Check sheet for the modelled part. Datum: model origin and axes. Units: mm. A direction names the side the tool comes from. Round coordinates to 2 decimals unless told otherwise and drop trailing zeros. Loops run counter-clockwise (first coordinate to the right, second up) from the corner with the lowest first, then second, coordinate; pieces in that order, holes last. Notation, with made-up numbers: (12, 32.25) -> (65, 32.25) arc R12 ccw to (65, 48.25) -> close; hole circle Ø7 at (51, 45.25). An arc over 180 degrees is marked (long way). One line per item, written item: value. Start each with the question number.
1. Go/stop test with flat-tipped pins: pin 1 (0.5 mm diameter, centred on y = 22, z = -42, fed in from +X); pin 2 (10 mm diameter, centred on y = 6, z = 71, fed in from +X); pin 3 (1.3 mm diameter, centred on y = 6, z = -42, fed in from +X). Record where each tip stops, or that it passes through.
2. Cross-section at A-A on y = 5.76. Count the separate pieces of the cut face and the enclosed holes in it, then the cut area to 3 significant figures.
3. Set-up check for faces 1 (the face through (67.25, 19.112, -37.995)), 2 (the face through (-0.912, 12, 22)), 3 (the face through (-2.131, 11, 22)), 4 (the face through (40, 14, -41.521)), 5 (the face through (67.869, 11, -36)): record each of +Z, -Z, +X, -X, +Y, -Y from which the full face is reachable in a straight line by a thin tool's end or side.
4. Material ranges on L1, parallel to Z at x = 3, y = 13.75; L2, parallel to X at y = 2.25, z = 83; L3, parallel to Y at x = 45.5, z = 32, recorded low to high.
5. Release check for a two-part mould opening along Z. For faces 6 (the face through (31, 11, 89.3)), 7 (the face through (67.869, 11, 83)), 8 (the face through (31, 12, 88.08)), 9 (the face through (25, 14, -42.74)) record: +Z half, -Z half, draft (parallel to the pull), parting line (faces both ways), or undercut.
6. Cross-section at C-C on x = 4. Record the cut outline in (y, z), then the cut area to 3 significant figures.
7. Cross-section at B-B on z = 32. Record the cut outline in (x, y).
from build123d import *

# Parameters (mm, degrees)
SKETCH2_W                    = 70
SKETCH2_H                    = 132.04
BASE_FLANGE1_DEPTH           = 1.2192
EDGE_FLANGE1_STRIP_W         = 6.3968
EDGE_FLANGE1_STRIP_H         = 1.2192
EDGE_FLANGE1_STRIP_CUT_DEPTH = 70
EDGE_FLANGE1_DEPTH           = 70
EDGE_FLANGE2_STRIP_W         = 6.3968
EDGE_FLANGE2_STRIP_H         = 1.2192
EDGE_FLANGE2_STRIP_CUT_DEPTH = 70
EDGE_FLANGE2_DEPTH           = 70
EDGE_FLANGE3_STRIP_W         = 6.3968
EDGE_FLANGE3_STRIP_H         = 1.2192
EDGE_FLANGE3_STRIP_CUT_DEPTH = 21.73
EDGE_FLANGE3_DEPTH           = 21.73
EDGE_FLANGE4_STRIP_W         = 6.3968
EDGE_FLANGE4_STRIP_H         = 1.2192
EDGE_FLANGE4_STRIP_CUT_DEPTH = 21.73
EDGE_FLANGE4_DEPTH           = 21.73
EDGE_FLANGE5_STRIP_W         = 6.3968
EDGE_FLANGE5_STRIP_H         = 1.2192
EDGE_FLANGE5_STRIP_CUT_DEPTH = 128.0816
EDGE_FLANGE5_DEPTH           = 128.0816
SKETCH24_W                   = 2.12
SKETCH24_H                   = 1.9792
CUT_EXTRUDE1_DEPTH           = 1.98
SKETCH29_W                   = 1.9792
SKETCH29_H                   = 2.12
CUT_EXTRUDE2_DEPTH           = 1.98
SKETCH30_W                   = 1.9792
SKETCH30_H                   = 1.9792
CUT_EXTRUDE3_DEPTH           = 1.98
SKETCH31_W                   = 1.9792
SKETCH31_H                   = 1.9792
CUT_EXTRUDE4_DEPTH           = 1.98
SKETCH34_W                   = 1.9792
SKETCH34_H                   = 1
CUT_EXTRUDE5_DEPTH           = 151.154943887
F_4_0MM_DOWEL_HOLE1_D        = 4
F_4_0MM_DOWEL_HOLE1_DEPTH    = 1.2192
CUT_EXTRUDE6_REACH           = 152.155
SKETCH38_W                   = 11
SKETCH38_H                   = 7.5
CUT_EXTRUDE7_REACH           = 152.155
SKETCH39_W                   = 11
SKETCH39_H                   = 7.5
CUT_EXTRUDE8_REACH           = 117.673
SKETCH40_W                   = 15
SKETCH40_H                   = 3
M2_TAPPED_HOLE1_D            = 1.6
CUT_EXTRUDE9_REACH           = 116.396
SKETCH41_W                   = 10
SKETCH41_H                   = 10
CUT_EXTRUDE10_REACH          = 152.155
SKETCH45_W                   = 21.5
SKETCH45_H                   = 8


# Sheet-metal steps are written as plain solids
with BuildPart() as part:
    # Sketch2 → Base-Flange1 (new body)
    with BuildSketch(Plane(origin=(0, 0, 0), x_dir=(1, 0, 0), z_dir=(0, 1, 0))):
        with Locations((32.868589744, -23.279615385)):
            Rectangle(SKETCH2_W, SKETCH2_H)
    extrude(amount=-BASE_FLANGE1_DEPTH)

    # Edge-Flange1 strip (across the edge) → Edge-Flange1 strip cut (cut)
    with BuildSketch(Plane(origin=(67.868589744, 0, -42.740384615), x_dir=(0, 0, 1), z_dir=(-1, 0, 0))):
        with Locations((-1.2192, -0.6096)):
            Rectangle(EDGE_FLANGE1_STRIP_W, EDGE_FLANGE1_STRIP_H)
    extrude(amount=EDGE_FLANGE1_STRIP_CUT_DEPTH, mode=Mode.SUBTRACT)

    # Edge-Flange1 section (across the edge) → Edge-Flange1 (add)
    with BuildSketch(Plane(origin=(67.868589744, 0, -42.740384615), x_dir=(0, 0, 1), z_dir=(-1, 0, 0))):
        with BuildLine():
            Line((0, 0.76), (0, 22.49))
            Line((0, 22.49), (1.2192, 22.49))
            Line((1.2192, 22.49), (1.2192, 0.76))
            ThreePointArc((1.2192, 0.76), (1.441798846, 0.222598846), (1.9792, 0))
            Line((1.9792, 0), (1.9792, -1.2192))
            ThreePointArc((1.9792, -1.2192), (0.579694259, -0.639505741), (0, 0.76))
        make_face()
    extrude(amount=EDGE_FLANGE1_DEPTH)

    # Edge-Flange2 strip (across the edge) → Edge-Flange2 strip cut (cut)
    with BuildSketch(Plane(origin=(-2.131410256, 0, 89.299615385), x_dir=(0, 0, -1), z_dir=(1, 0, 0))):
        with Locations((-1.2192, -0.6096)):
            Rectangle(EDGE_FLANGE2_STRIP_W, EDGE_FLANGE2_STRIP_H)
    extrude(amount=EDGE_FLANGE2_STRIP_CUT_DEPTH, mode=Mode.SUBTRACT)

    # Edge-Flange2 section (across the edge) → Edge-Flange2 (add)
    with BuildSketch(Plane(origin=(-2.131410256, 0, 89.299615385), x_dir=(0, 0, -1), z_dir=(1, 0, 0))):
        with BuildLine():
            Line((0, 0.76), (0, 22.49))
            Line((0, 22.49), (1.2192, 22.49))
            Line((1.2192, 22.49), (1.2192, 0.76))
            ThreePointArc((1.2192, 0.76), (1.441798846, 0.222598846), (1.9792, 0))
            Line((1.9792, 0), (1.9792, -1.2192))
            ThreePointArc((1.9792, -1.2192), (0.579694259, -0.639505741), (0, 0.76))
        make_face()
    extrude(amount=EDGE_FLANGE2_DEPTH)

    # Edge-Flange3 strip (across the edge) → Edge-Flange3 strip cut (cut)
    with BuildSketch(Plane(origin=(67.868589744, 0.76, -41.521184615), x_dir=(-1, 0, 0), z_dir=(0, 1, 0))):
        with Locations((-1.2192, -0.6096)):
            Rectangle(EDGE_FLANGE3_STRIP_W, EDGE_FLANGE3_STRIP_H)
    extrude(amount=EDGE_FLANGE3_STRIP_CUT_DEPTH, mode=Mode.SUBTRACT)

    # Edge-Flange3 section (across the edge) → Edge-Flange3 (add)
    with BuildSketch(Plane(origin=(67.868589744, 0.76, -41.521184615), x_dir=(-1, 0, 0), z_dir=(0, 1, 0))):
        with BuildLine():
            Line((0, 0.76), (0, 10))
            Line((0, 10), (1.2192, 10))
            Line((1.2192, 10), (1.2192, 0.76))
            ThreePointArc((1.2192, 0.76), (1.441798846, 0.222598846), (1.9792, 0))
            Line((1.9792, 0), (1.9792, -1.2192))
            ThreePointArc((1.9792, -1.2192), (0.579694259, -0.639505741), (0, 0.76))
        make_face()
    extrude(amount=EDGE_FLANGE3_DEPTH)

    # Edge-Flange4 strip (across the edge) → Edge-Flange4 strip cut (cut)
    with BuildSketch(Plane(origin=(67.868589744, 22.49, 88.080415385), x_dir=(-1, 0, 0), z_dir=(0, -1, 0))):
        with Locations((-1.2192, -0.6096)):
            Rectangle(EDGE_FLANGE4_STRIP_W, EDGE_FLANGE4_STRIP_H)
    extrude(amount=EDGE_FLANGE4_STRIP_CUT_DEPTH, mode=Mode.SUBTRACT)

    # Edge-Flange4 section (across the edge) → Edge-Flange4 (add)
    with BuildSketch(Plane(origin=(67.868589744, 22.49, 88.080415385), x_dir=(-1, 0, 0), z_dir=(0, -1, 0))):
        with BuildLine():
            Line((0, 0.76), (0, 10))
            Line((0, 10), (1.2192, 10))
            Line((1.2192, 10), (1.2192, 0.76))
            ThreePointArc((1.2192, 0.76), (1.441798846, 0.222598846), (1.9792, 0))
            Line((1.9792, 0), (1.9792, -1.2192))
            ThreePointArc((1.9792, -1.2192), (0.579694259, -0.639505741), (0, 0.76))
        make_face()
    extrude(amount=EDGE_FLANGE4_DEPTH)

    # Edge-Flange5 strip (across the edge) → Edge-Flange5 strip cut (cut)
    with BuildSketch(Plane(origin=(-2.131410256, 0, -40.761184615), x_dir=(1, 0, 0), z_dir=(0, 0, 1))):
        with Locations((-1.2192, -0.6096)):
            Rectangle(EDGE_FLANGE5_STRIP_W, EDGE_FLANGE5_STRIP_H)
    extrude(amount=EDGE_FLANGE5_STRIP_CUT_DEPTH, mode=Mode.SUBTRACT)

    # Edge-Flange5 section (across the edge) → Edge-Flange5 (add)
    with BuildSketch(Plane(origin=(-2.131410256, 0, -40.761184615), x_dir=(1, 0, 0), z_dir=(0, 0, 1))):
        with BuildLine():
            Line((0, 0.76), (0, 22.49))
            Line((0, 22.49), (1.2192, 22.49))
            Line((1.2192, 22.49), (1.2192, 0.76))
            ThreePointArc((1.2192, 0.76), (1.441798846, 0.222598846), (1.9792, 0))
            Line((1.9792, 0), (1.9792, -1.2192))
            ThreePointArc((1.9792, -1.2192), (0.579694259, -0.639505741), (0, 0.76))
        make_face()
    extrude(amount=EDGE_FLANGE5_DEPTH)

    # Sketch24 → Cut-Extrude1 (cut)
    with BuildSketch(Plane.XZ.offset(1.2192)):
        with Locations((66.808589744, 88.310015385)):
            Rectangle(SKETCH24_W, SKETCH24_H)
    extrude(amount=-CUT_EXTRUDE1_DEPTH, mode=Mode.SUBTRACT)

    # Sketch29 → Cut-Extrude2 (cut)
    with BuildSketch(Plane.XZ.offset(1.2192)):
        with Locations((-1.141810256, 88.380415385)):
            Rectangle(SKETCH29_W, SKETCH29_H)
    extrude(amount=-CUT_EXTRUDE2_DEPTH, mode=Mode.SUBTRACT)

    # Sketch30 → Cut-Extrude3 (cut)
    with BuildSketch(Plane.XZ.offset(1.2192)):
        with Locations((-1.141810256, -41.750784615)):
            Rectangle(SKETCH30_W, SKETCH30_H)
    extrude(amount=-CUT_EXTRUDE3_DEPTH, mode=Mode.SUBTRACT)

    # Sketch31 → Cut-Extrude4 (cut)
    with BuildSketch(Plane.XZ.offset(1.2192)):
        with Locations((66.878989744, -41.750784615)):
            Rectangle(SKETCH31_W, SKETCH31_H)
    extrude(amount=-CUT_EXTRUDE4_DEPTH, mode=Mode.SUBTRACT)

    # Sketch34 → Cut-Extrude5 (cut, through all)
    with BuildSketch(Plane.XY.offset(89.299615385)):
        with Locations((66.878989744, 21.99)):
            Rectangle(SKETCH34_W, SKETCH34_H)
    extrude(amount=-CUT_EXTRUDE5_DEPTH, mode=Mode.SUBTRACT)

    # Ø4.0mm Dowel Hole1
    with Locations(Plane(origin=(67.868589744, 0, 0), x_dir=(0, 0, -1), z_dir=(1, 0, 0))):
        with Locations((-83.080415385, 17.76), (-83.080415385, 5.76), (36.521184615, 17.76), (36.521184615, 5.76)):
            Hole(F_4_0MM_DOWEL_HOLE1_D / 2, depth=F_4_0MM_DOWEL_HOLE1_DEPTH)

    # Sketch38 → Cut-Extrude6 (cut, up to next)
    with BuildSketch(Plane.XY.offset(89.299615385), mode=Mode.PRIVATE) as cut_extrude6_sk1:
        with Locations((22.088589744, 17.74)):
            Rectangle(SKETCH38_W, SKETCH38_H)
    cut_extrude6_tool1 = extrude(cut_extrude6_sk1.sketch, amount=-CUT_EXTRUDE6_REACH, mode=Mode.PRIVATE) & part.part
    add(cut_extrude6_tool1.solids().sort_by_distance((22.08859, 17.74, 89.299615))[0], mode=Mode.SUBTRACT)

    # Sketch39 → Cut-Extrude7 (cut, up to next)
    with BuildSketch(Plane(origin=(0, 0, -42.740384615), x_dir=(-1, 0, 0), z_dir=(0, 0, -1)), mode=Mode.PRIVATE) as cut_extrude7_sk1:
        with Locations((-31.338589744, 17.09)):
            Rectangle(SKETCH39_W, SKETCH39_H)
    cut_extrude7_tool1 = extrude(cut_extrude7_sk1.sketch, amount=-CUT_EXTRUDE7_REACH, mode=Mode.PRIVATE) & part.part
    add(cut_extrude7_tool1.solids().sort_by_distance((31.33859, 17.09, -42.740385))[0], mode=Mode.SUBTRACT)

    # Sketch40 → Cut-Extrude8 (cut, up to next)
    with BuildSketch(Plane.ZY.offset(2.131410256), mode=Mode.PRIVATE) as cut_extrude8_sk1:
        with Locations((51.420415385, 18.24)):
            Rectangle(SKETCH40_W, SKETCH40_H)
    cut_extrude8_tool1 = extrude(cut_extrude8_sk1.sketch, amount=-CUT_EXTRUDE8_REACH, mode=Mode.PRIVATE) & part.part
    add(cut_extrude8_tool1.solids().sort_by_distance((-2.13141, 18.24, 51.420415))[0], mode=Mode.SUBTRACT)

    # M2 Tapped Hole1 (through all)
    with Locations(Plane(origin=(0, 0, 0), x_dir=(1, 0, 0), z_dir=(0, 1, 0))):
        with Locations((24.618589744, 24.431184615), (41.118589744, 24.431184615), (41.118589744, -10.568815385), (24.618589744, -10.568815385)):
            Hole(M2_TAPPED_HOLE1_D / 2)

    # Sketch41 → Cut-Extrude9 (cut, up to next)
    with BuildSketch(Plane(origin=(0, 0, 0), x_dir=(1, 0, 0), z_dir=(0, 1, 0)), mode=Mode.PRIVATE) as cut_extrude9_sk1:
        with Locations((32.868589744, -10.568815385)):
            Rectangle(SKETCH41_W, SKETCH41_H)
    cut_extrude9_tool1 = extrude(cut_extrude9_sk1.sketch, amount=-CUT_EXTRUDE9_REACH, mode=Mode.PRIVATE) & part.part
    add(cut_extrude9_tool1.solids().sort_by_distance((32.86859, 0, 10.568815))[0], mode=Mode.SUBTRACT)

    # Sketch45 → Cut-Extrude10 (cut, up to next)
    with BuildSketch(Plane(origin=(0, 0, -42.740384615), x_dir=(-1, 0, 0), z_dir=(0, 0, -1)), mode=Mode.PRIVATE) as cut_extrude10_sk1:
        with Locations((-32.868589744, 7.8608)):
            Rectangle(SKETCH45_W, SKETCH45_H)
    cut_extrude10_tool1 = extrude(cut_extrude10_sk1.sketch, amount=-CUT_EXTRUDE10_REACH, mode=Mode.PRIVATE) & part.part
    add(cut_extrude10_tool1.solids().sort_by_distance((32.86859, 7.8608, -42.740385))[0], mode=Mode.SUBTRACT)


solid = part.part
Taken from the geometry:
1. pin 1: stops at x = 65.89
1. pin 2: stops at x = -0.91
1. pin 3: stops at x = 67.78
2. separate pieces: 6
2. enclosed holes: 0
2. area: 314 mm2
3. face 1: +X
3. face 2: +Y
3. face 3: +Z, -Z, -X, +Y, -Y
3. face 4: -X, +Y
3. face 5: +Z, -Z, +X, +Y, -Y
4. L1: z = -42.74 to -41.52, 88.08 to 89.3
4. L2: x = -2.13 to -0.91, 66.65 to 67.87
4. L3: y = -1.22 to 0
5. face 6: +Z half
5. face 7: draft
5. face 8: undercut
5. face 9: -Z half
6. outline: (-1.22, -40.76) arc R1.98 ccw to (0.76, -42.74) -> (22.49, -42.74) -> (22.49, -41.52) -> (0.76, -41.52) arc R0.76 cw to (0, -40.76) -> (0, 87.32) arc R0.76 cw to (0.76, 88.08) -> (22.49, 88.08) -> (22.49, 89.3) -> (0.76, 89.3) arc R1.98 ccw to (-1.22, 87.32) -> close
6. area: 214 mm2
7. outline: (-2.13, 0.76) arc R1.98 ccw to (-0.15, -1.22) -> (67.87, -1.22) -> (67.87, 0) -> (-0.15, 0) arc R0.76 cw to (-0.91, 0.76) -> (-0.91, 22.49) -> (-2.13, 22.49) -> close
